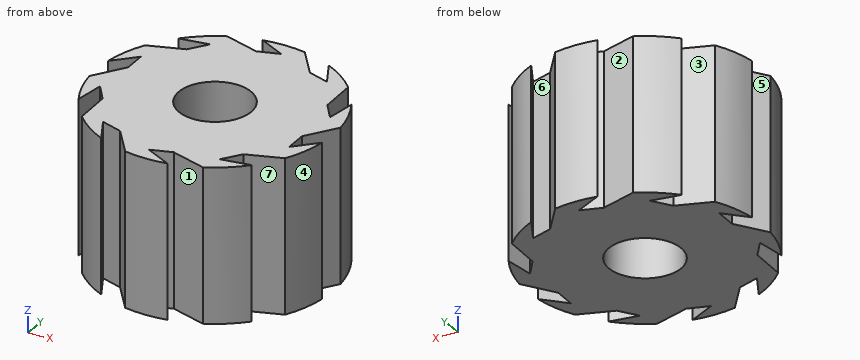
from build123d import *

# Parameters (mm, degrees)
F2_R            = 9.525
F2_R_2          = 2.921
F3_DEPTH        = 12.446
F5_DEPTH        = 12.446
F5_COPIES_COUNT = 10


# Not quite as in the source:
# - a pattern or mirror of a feature is missing from the dataset's text; its kind, count and spacing are read off the source's solid


with BuildPart() as f3:
    # F2 (on Top) → F3 (new body)
    with BuildSketch(Plane.XY):
        Circle(F2_R)
        Circle(F2_R_2, mode=Mode.SUBTRACT)
    extrude(amount=F3_DEPTH)

    # F4 (on face) → F5 (cut, through all)
    with BuildSketch(Plane.XY.offset(12.446)):
        Polygon((9.525, -1.27), (9.525, 1.27), (7.747, -1.269247156), (7.747, -3.048), align=None)
    f5 = extrude(amount=-F5_DEPTH, mode=Mode.SUBTRACT)

    # F5_copies: F5 ×10 about axis
    f5_copies_axis = Axis((0, 0, 0), (0, 0, 1))
    for i in range(1, F5_COPIES_COUNT):
        add(f5.rotate(f5_copies_axis, i * 360 / F5_COPIES_COUNT), mode=Mode.SUBTRACT)


solid = f3.part
Here's how the part is built. I have some questions about the finished solid (model axes, mm). Face numbers are marked on the shaded views. A direction names the side the tool comes from. Give positions to 0.01 mm unless a question says otherwise; leave off trailing zeros. Loops run counter-clockwise (first coordinate to the right, second up) from the corner with the lowest first, then second, coordinate; pieces in that order, holes last. Notation, with made-up numbers: (70.5, 34) -> (83.5, 34) arc R14 cw to (83.5, 53) -> close; hole circle Ø6 at (51, 18.5). An arc over 180 degrees is marked (long way). Answer as a JSON object with one key per item and string values. Group by question number.
Item 1: I need wall thicknesses on L1, parallel to Y at x = -4.75, z = 8.5; L2, parallel to Y at x = -1.25, z = 7.5; L3, parallel to Y at x = 0, z = 7.75 (3 decimals). Which ranges of each line are inside material? Lowest first, please.
Item 2: Imagine slicing it at A-A on y = 0. Write out the boundary of the cut face in (x, z).
Item 3: Will these pins go through, and if not, where does the flat tip stop? pin 1 (2 mm diameter, centred on y = -1.5, z = 5.5, fed in from +X); pin 2 (6 mm diameter, centred on x = -3.5, z = 8.5, fed in from +Y); pin 3 (3.5 mm diameter, centred on x = 0, y = 0, fed in from +Z); pin 4 (2 mm diameter, centred on y = 2, z = 3.5, fed in from -X).
Item 4: Thinking about a two-plate mould opening in X: for the marked faces 1, 2, 3 and 4, which applies, pulls with the +X half, pulls with the -X half, needs draft (parallel to the pull), parting line crosses it, or undercut?
Item 5: Imagine slicing it at B-B on x = 0. Write out the boundary of the cut face in (y, z) (3 decimals).
Item 6: On a 3-axis mill with a long thin cutter (end or side, diameter ignored), from which of +Z, -Z, +X, -X, +Y, -Y can I reach the whole of each face in a straight line? I mean the marked faces 5, 6 and 7. Say none if no direction works.
Answer list:
{
 "1": {"L1": "y = -8.26 to -7.49, -6.6 to 6.64, 6.98 to 8.26", "L2": "y = -9.44 to -2.64, 2.64 to 7.78, 9.2 to 9.44", "L3": "y = -9.525 to -8.567, -8.146 to -2.921, 2.921 to 8.146, 8.567 to 9.525"},
 "2": {"outline": "(-8.64, 0) -> (-2.92, 0) -> (-2.92, 12.45) -> (-8.64, 12.45) -> close; (2.92, 0) -> (8.64, 0) -> (8.64, 12.45) -> (2.92, 12.45) -> close"},
 "3": {"pin 1": "stops at x = 9.43", "pin 2": "stops at y = 9.51", "pin 3": "passes through", "pin 4": "stops at x = -9.43"},
 "4": {"face 1": "undercut", "face 2": "undercut", "face 3": "pulls with the -X half", "face 4": "pulls with the +X half"},
 "5": {"outline": "(-9.525, 0) -> (-8.567, 0) -> (-8.567, 12.446) -> (-9.525, 12.446) -> close; (-8.146, 0) -> (-2.921, 0) -> (-2.921, 12.446) -> (-8.146, 12.446) -> close; (2.921, 0) -> (8.146, 0) -> (8.146, 12.446) -> (2.921, 12.446) -> close; (8.567, 0) -> (9.525, 0) -> (9.525, 12.446) -> (8.567, 12.446) -> close"},
 "6": {"face 5": "+Z, -Z, -X", "face 6": "+Z, -Z", "face 7": "+Z, -Z, +X"}
}
